Work out the finished part from the listing and answer in its coordinate system (mm). A direction names the side the tool comes from. Coordinates: 2 decimals unless noted, no trailing zeros. Order: outer loops, then holes, each group sorted by start corner. A loop starts at its lowest first (then second) coordinate and runs counter-clockwise, first axis right, second up. Notation, with made-up numbers: (-0.75, -2) -> (32.25, -2) arc R27 cw to (32.25, 37) -> close; hole circle Ø2 at (86.5, 56.5). An arc over 180 degrees is marked (long way). Write item = value, one per line. Start each with the question number.
Q1. For a pull along Z with two mould halves and no side action, classify faces 1 (the cylindrical face through (2, -81, 0)), 2 (the flat face through (33, 4, -37)), 3 (the cylindrical face through (-46.798, -0.056, -29.836)) as +Z half, -Z half, draft (parallel to the pull), parting line (faces both ways), or undercut.
Q2. The part is cut by section B-B, the plane z = -40.5. Determine the outline of the cut face in (x, y), plus the area to 3 significant figures.
Q3. The part is cut by section C-C, the plane y = 6. Determine the outline of the cut face in (x, z).
Q4. The part is cut by section A-A, the plane x = 32.5. Determine the outline of the cut face in (y, z).
Q5. Straight lines are drawn through the part: L1, parallel to X at y = -81, z = 0; L2, parallel to X at y = -17.75, z = 0; L3, parallel to Z at x = 23.5, y = 17. For each, find the intervals that lie inside material, in ascending order. Write a range as from..to.
Q6. Which of the six approach directions +Z, -Z, +X, -X, +Y, -Y give full straight-line access (tool end or side, diameter ignored) to faces 4 (the cylindrical face through (27.686, -14.79, 36.107)), 5 (the flat face through (0, -4, 50)), 6 (the cylindrical face through (-9.54, 61.63, 3)), 7 (the flat face through (0, 73.5, 0))?
Q7. Flat-ended cylindrical pins translate along their axes: pin 1 (1 mm diameter, centred on y = -65.5, z = 15.5, fed in from -X); pin 2 (1 mm diameter, centred on x = 35.5, y = 28.5, fed in from -Z); pin 3 (5 mm diameter, centred on x = 38, y = -50.5, fed in from -Z). Find the tip coordinate at first contact, or state that the pin passes through.
```python
from build123d import *

# Parameters (mm, degrees)
SKETCH2_R           = 10
BOSS_EXTRUDE1_DEPTH = 26
SKETCH3_R           = 5
SKETCH3_R_2         = 2
BOSS_EXTRUDE2_DEPTH = 5
FILLET1_R           = 2
FILLET3_R           = 1


with BuildPart() as part:
    # Sketch1 → Revolve2 (revolve)
    with BuildSketch(Plane.XY, mode=Mode.PRIVATE) as revolve2_sk:
        with BuildLine():
            Line((-55.5, -4), (-49.5, -4))
            Line((-49.5, -4), (-49.5, -30))
            ThreePointArc((-49.5, -30), (-35.001785669, -65.001785669), (0, -79.5))
            Line((0, -79.5), (0, -75.5))
            ThreePointArc((0, -75.5), (-32.173358544, -62.173358544), (-45.5, -30))
            Line((-45.5, -30), (-45.5, 0))
            ThreePointArc((-45.5, 0), (-32.173358544, 32.173358544), (0, 45.5))
            Line((0, 45.5), (0, 49.5))
            ThreePointArc((0, 49.5), (-33.557785982, 36.388528412), (-49.338119137, 4))
            Line((-49.338119137, 4), (-55.5, 4))
            Line((-55.5, 4), (-55.5, 0))
            Line((-55.5, 0), (-55.5, -4))
        make_face()
    revolve(revolve2_sk.sketch.rotate(Axis((0, -85.95, 0), (0, 1, 0)), 270), axis=Axis((0, -85.95, 0), (0, 1, 0)))

    # Sketch2 → Boss-Extrude1 (add)
    with BuildSketch(Plane(origin=(0, 47.5, 0), x_dir=(1, 0, 0), z_dir=(0, 1, 0))):
        with Locations(Location((0, 0, 0), (0, 0, 180))):
            Circle(SKETCH2_R)
    extrude(amount=BOSS_EXTRUDE1_DEPTH)

    # Sketch3 → Boss-Extrude2 (add)
    with BuildSketch(Plane(origin=(0, -77.5, 0), x_dir=(-1, 0, 0), z_dir=(0, -1, 0))):
        with Locations(Location((0, 0, 0), (0, 0, 270))):
            Circle(SKETCH3_R)
        with Locations(Location((0, 0, 0), (0, 0, 270))):
            Circle(SKETCH3_R_2, mode=Mode.SUBTRACT)
    extrude(amount=BOSS_EXTRUDE2_DEPTH)

    # Fillet1
    fillet1_edges = [part.edges().sort_by_distance(p)[0] for p in [
        (7.071067812, 48.479377059, 7.071067812),
    ]]
    fillet(fillet1_edges, radius=FILLET1_R)

    # Fillet3
    fillet3_edges = [part.edges().sort_by_distance(p)[0] for p in [
        (-4.999999999, -79.246827309, 0),
    ]]
    fillet(fillet3_edges, radius=FILLET3_R)


solid = part.part
```
Model answer:
q1.face_1 = undercut
q1.face_2 = draft
q1.face_3 = parting line
q2.outline = (-37.95, -4) -> (-28.46, -4) -> (-28.46, -30) arc R28.46 ccw to (28.46, -30) -> (28.46, -4) -> (37.95, -4) -> (37.95, 4) -> (28.18, 4) arc R28.46 ccw to (-28.18, 4) -> (-37.95, 4) -> close; hole (-20.74, -30) arc R20.74 ccw to (20.74, -30) -> (20.74, 0) arc R20.74 ccw to (-20.74, 0) -> close
q2.area = 1,810 mm2
q3.outline = circle Ø98.27 at (0, 0); hole circle Ø90.21 at (0, 0)
q4.outline = (-30, -37.34) -> (-4, -37.34) -> (-4, -44.99) -> (4, -44.99) -> (4, -37.12) arc R37.34 ccw to (4, 37.12) -> (4, 44.99) -> (-4, 44.99) -> (-4, 37.34) -> (-30, 37.34) arc R37.34 ccw to start; hole (-30, -31.84) -> (0, -31.84) arc R31.84 ccw to (0, 31.84) -> (-30, 31.84) arc R31.84 ccw to start
q5.L1 = -5..-2, 2..5
q5.L2 = -49.5..-45.5, 45.5..49.5
q5.L3 = -40.11..-35.06, 35.06..40.11
q6.face_4 = none
q6.face_5 = -Y
q6.face_6 = +Y
q6.face_7 = +Z, -Z, +X, -X, +Y
q7.pin_1 = -31.44
q7.pin_2 = -20.57
q7.pin_3 = -28.21
